from build123d import *

# Parameters (mm, degrees)
BOSS_EXTRUDE1_DEPTH      = 8.1
BOSS_EXTRUDE1_DEPTH_BACK = 8.1
BOSS_EXTRUDE5_REACH      = 25.5
SKETCH2_R                = 8
SKETCH3_R                = 2.5
BOSS_EXTRUDE6_DEPTH      = 0.5
SKETCH4_R                = 2.4
BOSS_EXTRUDE7_DEPTH      = 20
SKETCH8_R                = 2
BOSS_EXTRUDE8_DEPTH      = 19
SKETCH11_R               = 2
SKETCH11_R_2             = 1.75
BOSS_EXTRUDE10_DEPTH     = 18
CUT_EXTRUDE1_REACH       = 22
SKETCH13_R               = 1.5


with BuildPart() as part:
    # Sketch1 → Boss-Extrude1 (new body, two sides)
    with BuildSketch(Plane.XY) as boss_extrude1_sk:
        with BuildLine():
            Line((-10, 12.5), (10, 12.5))
            Line((10, 12.5), (10, -10.5))
            ThreePointArc((10, -10.5), (9.414213562, -11.914213562), (8, -12.5))
            Line((8, -12.5), (-8, -12.5))
            ThreePointArc((-8, -12.5), (-9.414213562, -11.914213562), (-10, -10.5))
            Line((-10, -10.5), (-10, 12.5))
        make_face()
        with BuildLine():
            Line((-8.5, 11), (-8.5, -10.5))
            ThreePointArc((-8.5, -10.5), (-8.353553391, -10.853553391), (-8, -11))
            Line((-8, -11), (8, -11))
            ThreePointArc((8, -11), (8.353553391, -10.853553391), (8.5, -10.5))
            Line((8.5, -10.5), (8.5, 11))
            Line((8.5, 11), (-8.5, 11))
        make_face(mode=Mode.SUBTRACT)
    extrude(amount=BOSS_EXTRUDE1_DEPTH)
    extrude(boss_extrude1_sk.sketch, amount=-BOSS_EXTRUDE1_DEPTH_BACK)

    # Sketch2 → Boss-Extrude5 (add, up to next)
    with BuildSketch(Plane(origin=(0, -11, 0), x_dir=(1, 0, 0), z_dir=(0, 1, 0)), mode=Mode.PRIVATE) as boss_extrude5_sk1:
        Circle(SKETCH2_R)
    boss_extrude5_tool1 = extrude(boss_extrude5_sk1.sketch, amount=BOSS_EXTRUDE5_REACH, mode=Mode.PRIVATE) - part.part
    add(boss_extrude5_tool1.solids().sort_by_distance((0, -11, 0))[0])

    # Sketch3 → Boss-Extrude6 (add)
    with BuildSketch(Plane.XZ.offset(12.5)):
        Circle(SKETCH3_R)
    extrude(amount=BOSS_EXTRUDE6_DEPTH)

    # Sketch4 → Boss-Extrude7 (add)
    with BuildSketch(Plane(origin=(0, 12.5, 0), x_dir=(1, 0, 0), z_dir=(0, 1, 0))):
        with BuildLine():
            ThreePointArc((-5.405212541, 2.604549364), (-6, 0), (-5.405212541, -2.604549364))
            ThreePointArc((-5.405212541, -2.604549364), (-7.12383297, -7.12383297), (-2.604549364, -5.405212541))
            ThreePointArc((-2.604549364, -5.405212541), (0, -6), (2.604549364, -5.405212541))
            ThreePointArc((2.604549364, -5.405212541), (7.12383297, -7.12383297), (5.405212541, -2.604549364))
            ThreePointArc((5.405212541, -2.604549364), (6, 0), (5.405212541, 2.604549364))
            ThreePointArc((5.405212541, 2.604549364), (7.12383297, 7.12383297), (2.604549364, 5.405212541))
            ThreePointArc((2.604549364, 5.405212541), (0, 6), (-2.604549364, 5.405212541))
            ThreePointArc((-2.604549364, 5.405212541), (-7.12383297, 7.12383297), (-5.405212541, 2.604549364))
        make_face()
        with Locations((-5.25, 5.25)):
            Circle(SKETCH4_R, mode=Mode.SUBTRACT)
        with Locations((5.25, 5.25)):
            Circle(SKETCH4_R, mode=Mode.SUBTRACT)
        with Locations((5.25, -5.25)):
            Circle(SKETCH4_R, mode=Mode.SUBTRACT)
        with Locations((-5.25, -5.25)):
            Circle(SKETCH4_R, mode=Mode.SUBTRACT)
    extrude(amount=BOSS_EXTRUDE7_DEPTH)

    # Sketch6 → Revolve1 (revolve)
    with BuildSketch(Plane.XY):
        Polygon((1.25, 32.5), (1.25, 43), (2, 43), (2, 38.5), (2.4, 37.5), (2, 37.5), (2, 32.5), align=None)
    revolve(axis=Axis((0, 32.5, 0), (0, 1, 0)))

    # Sketch8 → Boss-Extrude8 (add)
    with BuildSketch(Plane(origin=(0, 12.5, 0), x_dir=(1, 0, 0), z_dir=(0, 1, 0))):
        with Locations((-5.25, 5.25)):
            Circle(SKETCH8_R)
        with Locations((5.25, 5.25)):
            Circle(SKETCH8_R)
        with Locations((5.25, -5.25)):
            Circle(SKETCH8_R)
        with Locations((-5.25, -5.25)):
            Circle(SKETCH8_R)
    extrude(amount=BOSS_EXTRUDE8_DEPTH)

    # Sketch11 → Boss-Extrude10 (add)
    with BuildSketch(Plane.XY):
        with Locations((0, 19.5)):
            Circle(SKETCH11_R)
        with Locations((0, 19.5)):
            Circle(SKETCH11_R_2, mode=Mode.SUBTRACT)
    extrude(amount=BOSS_EXTRUDE10_DEPTH)

    # Sketch12 → Revolve2 (revolve)
    with BuildSketch(Plane(origin=(0, 0, 0), x_dir=(0, 0, -1), z_dir=(1, 0, 0))):
        Polygon((-14, 21.5), (-13, 22), (-13, 21.5), align=None)
    revolve(axis=Axis((0, 19.5, 18), (0, 0, -1)))

    # Sketch13 → Cut-Extrude1 (cut, up to next)
    with BuildSketch(Plane.ZY.offset(10), mode=Mode.PRIVATE) as cut_extrude1_sk1:
        with Locations((-5.1, 7.25)):
            Circle(SKETCH13_R)
    cut_extrude1_tool1 = extrude(cut_extrude1_sk1.sketch, amount=-CUT_EXTRUDE1_REACH, mode=Mode.PRIVATE) & part.part
    add(cut_extrude1_tool1.solids().sort_by_distance((-10, 7.25, -5.1))[0], mode=Mode.SUBTRACT)
    # Sketch13 → Cut-Extrude1 (cut, up to next)
    with BuildSketch(Plane.ZY.offset(10), mode=Mode.PRIVATE) as cut_extrude1_sk2:
        with Locations((5.1, -7.25)):
            Circle(SKETCH13_R)
    cut_extrude1_tool2 = extrude(cut_extrude1_sk2.sketch, amount=-CUT_EXTRUDE1_REACH, mode=Mode.PRIVATE) & part.part
    add(cut_extrude1_tool2.solids().sort_by_distance((-10, -7.25, 5.1))[0], mode=Mode.SUBTRACT)


solid = part.part
Input: part model. Units: mm. Frame: model coordinates. A direction names the side the tool comes from. Coordinates: 2 decimals unless noted, no trailing zeros. Loops run counter-clockwise (first coordinate to the right, second up) from the corner with the lowest first, then second, coordinate; pieces in that order, holes last. Notation, with made-up numbers: (-16.75, -29.75) - (7.25, -29.75) arc R13 cw to (7.25, -24.75) - close; hole circle Ø9 at (47.25, 0). An arc over 180 degrees is marked (long way). Answer in a Markdown table with one row per item. Add a question column.
Item 1: Line query: line 1 along Z through (x, y) = (5.25, 20); line 2 along Y through (x, z) = (-3.75, 8). Output: solid intervals per line, ascending. Write a range as [from, to].
Item 2: Mould query, pull axis X, two halves, no side actions, for faces 5 (the flat face through (-1, 37.5, -2)), 6 (the cylindrical face through (0, 35, 2)), 7 (the cylindrical face through (-9.4, -11.93, 0.11)), 8 (the cylindrical face through (7.54, 22.36, 4.53)). Classes: released by +X, released by -X, zero draft, split by the parting line, or undercut.
Item 3: Access query for faces 1 (the flat face through (-1, 43, -1)), 2 (the flat face through (-5, 31.5, 5)), 3 (the cylindrical face through (-9.26, -8.58, 5.79)), 4 (the flat face through (-8.5, 0, 0)). Directions: +Z, -Z, +X, -X, +Y, -Y. A direction counts if a zero-diameter tool reaches every point of the face in a straight line with its end or side. Return the directions, or none.
Item 4: Section query C-C on z = 14.75. Return the cut outline in (x, y).
Item 5: Section query B-B on y = 2.5. Return the cut outline in (x, z), then the cut area to 3 significant figures.
Item 6: Section query D-D on y = 34.5. Return the cut outline in (x, z), then the cut area to 3 significant figures.
Item 7: Section query A-A on y = -7.25. Return the cut outline in (x, z).
Item 8: Contact query for flat-ended pins moving along their axis: P1, Ø1.5, axis at x = -3, y = 24.5, coming from the +Z side; P2, Ø12, axis at x = -6, y = 5.5, coming from the +Z side; P3, Ø6, axis at x = 3.5, z = -1.5, coming from the -Y side; P4, Ø2.5, axis at x = 4, z = -5.5, coming from the +Y side. Output: stop coordinate, or through.
Recorded:
| question | item | result |
|---|---|---|
| 1 | line 1 | [-7.9, -7.65], [-7.25, -3.25], [-2.85, 2.85], [3.25, 7.25], [7.65, 7.9] |
| 1 | line 2 | [-12.5, -11], [11, 12.5] |
| 2 | face 5 | zero draft |
| 2 | face 6 | split by the parting line |
| 2 | face 7 | released by -X |
| 2 | face 8 | undercut |
| 3 | face 1 | +Z, -Z, +X, -X, +Y |
| 3 | face 2 | +Y |
| 3 | face 3 | -X |
| 3 | face 4 | +Z, -Z |
| 4 | outline | circle Ø4 at (0, 19.5); hole circle Ø3.5 at (0, 19.5) |
| 5 | outline | (-10, -8.1) - (-8.5, -8.1) - (-8.5, 8.1) - (-10, 8.1) - close; circle Ø16 at (0, 0); (8.5, -8.1) - (10, -8.1) - (10, 8.1) - (8.5, 8.1) - close |
| 5 | area | 250 mm^2 |
| 6 | outline | circle Ø4 at (0, 0); hole circle Ø2.5 at (0, 0) |
| 6 | area | 7.66 mm^2 |
| 7 | outline | (-10, -8.1) - (-8.5, -8.1) - (-8.5, 3.6) - (-10, 3.6) - close; (-10, 6.6) - (-8.5, 6.6) - (-8.5, 8.1) - (-10, 8.1) - close; circle Ø16 at (0, 0); (8.5, -8.1) - (10, -8.1) - (10, 8.1) - (8.5, 8.1) - close |
| 8 | P1 | z = 7.43 |
| 8 | P2 | z = 8.1 |
| 8 | P3 | y = -13 |
| 8 | P4 | y = 32.5 |
